Geometry: final body of the model. Coordinates: model frame, mm. Give positions to 0.01 mm unless a question says otherwise; leave off trailing zeros. Loops run counter-clockwise (first coordinate to the right, second up) from the corner with the lowest first, then second, coordinate; pieces in that order, holes last.
```python
from build123d import *

# Parameters (mm, degrees)
SKETCH1_W           = 650
SKETCH1_H           = 500
SKETCH1_W_2         = 450
SKETCH1_H_2         = 422
BOSS_EXTRUDE1_DEPTH = 13
SKETCH2_W           = 450
SKETCH2_H           = 10
CUT_EXTRUDE1_DEPTH  = 13
SHELL1_T            = -1
SKETCH3_R           = 4
BOSS_EXTRUDE2_DEPTH = 2
LPATTERN1_COUNT     = 2
LPATTERN1_PITCH     = 45


with BuildPart() as part:
    # Sketch1 → Boss-Extrude1 (new body)
    with BuildSketch(Plane.XY):
        Rectangle(SKETCH1_W, SKETCH1_H)
        Rectangle(SKETCH1_W_2, SKETCH1_H_2, mode=Mode.SUBTRACT)
    extrude(amount=BOSS_EXTRUDE1_DEPTH)

    # Sketch2 → Cut-Extrude1 (cut)
    with BuildSketch(Plane(origin=(0, 0, 0), x_dir=(-1, 0, 0), z_dir=(0, 0, -1))):
        with Locations((0, -216)):
            Rectangle(SKETCH2_W, SKETCH2_H)
    extrude(amount=-CUT_EXTRUDE1_DEPTH, mode=Mode.SUBTRACT)

    # Shell1
    shell1_openings = [part.faces().sort_by_distance(p)[0] for p in [
        (0, -241.799390267, 13),
        (-225, -5, 6.5),
        (225, -5, 6.5),
        (0, 211, 6.5),
        (0, -221, 6.5),
    ]]
    offset(amount=SHELL1_T, openings=shell1_openings, kind=Kind.INTERSECTION)

    # Sketch3 → Boss-Extrude2 (add)
    with BuildSketch(Plane.XY.offset(1)):
        with Locations((-240.106920594, 180)):
            Circle(SKETCH3_R)
    boss_extrude2 = extrude(amount=BOSS_EXTRUDE2_DEPTH)

    # LPattern1: Boss-Extrude2 ×2
    with Locations(*[(0, -i * LPATTERN1_PITCH, 0) for i in range(1, LPATTERN1_COUNT)]):
        add(boss_extrude2)


solid = part.part
```
Q1. Pin query (flat end, axial travel): pin 1 Ø9 at (x, y) = (-241.5, 133.5) entering from +Z. Return the tip coordinate at first contact, or that it passes through.
Q2. Section query B-B, the plane x = -191. Return loops of the section in (y, z).
Q3. Mould query, pull axis X, two halves, no side actions, for faces 1 (the face through (-325, -3, 6)), 2 (the face through (-2, 241, 1)), 3 (the face through (325, -3, 6)). Classes: +X half, -X half, draft (parallel to the pull), parting line (faces both ways), or undercut.
Q4. Material intervals for probe 1 along Y at (x, z) = (98, 12); probe 2 along Y at (x, z) = (189, 0.75); probe 3 along X at (y, z) = (-91, 8.5), sorted ascending.
Q5. Section query A-A, the plane y = 123.5. Return loops of the section in (x, z).
Resolved:
1. pin 1: stops at z = 3
2. outline: (-250, 0) - (-221, 0) - (-221, 1) - (-249, 1) - (-249, 13) - (-250, 13) - close; (211, 0) - (250, 0) - (250, 13) - (249, 13) - (249, 1) - (211, 1) - close
3. face 1: -X half
3. face 2: undercut
3. face 3: +X half
4. probe 1: y = -250 to -249, 249 to 250
4. probe 2: y = -250 to -221, 211 to 250
4. probe 3: x = -325 to -324, 324 to 325
5. outline: (-325, 0) - (-225, 0) - (-225, 1) - (-324, 1) - (-324, 13) - (-325, 13) - close; (225, 0) - (325, 0) - (325, 13) - (324, 13) - (324, 1) - (225, 1) - close
